The model under review builds one solid part; all positions refer to its coordinate system, in mm. A direction names the side the tool comes from. Coordinates: 2 decimals unless noted, no trailing zeros. Loops run counter-clockwise (first coordinate to the right, second up) from the corner with the lowest first, then second, coordinate; pieces in that order, holes last. Notation, with made-up numbers: M 35.5,20 L 93.5,20 A25 ccw 93.5,46 Z; hole C -17,24.5 d8. An arc over 180 degrees is marked long. Return JSON: item names as keys, results as strings.
```python
from build123d import *

# Parameters (mm, degrees)
F0_W     = 1000
F0_H     = 600
F1_DEPTH = 25
F2_W     = 960
F2_H     = 560
F3_DEPTH = 400
F4_W     = 940
F4_H     = 540
F5_DEPTH = 380
F6_W     = 25
F6_H     = 25
F7_DEPTH = 500
F8_R     = 25
F9_DEPTH = 100


with BuildPart() as f1:
    # F0 (on Top) → F1 (new body)
    with BuildSketch(Plane.XY):
        Rectangle(F0_W, F0_H)
    extrude(amount=F1_DEPTH)

    # F2 (on face) → F3 (join)
    with BuildSketch(Plane.XY.offset(25)):
        Rectangle(F2_W, F2_H)
    extrude(amount=F3_DEPTH)

    # F4 (on face) → F5 (cut)
    with BuildSketch(Plane(origin=(0, 0, 0), x_dir=(1, 0, 0), z_dir=(0, 0, -1))):
        Rectangle(F4_W, F4_H)
    extrude(amount=-F5_DEPTH, mode=Mode.SUBTRACT)

    # F6 (on face) → F7 (join)
    with BuildSketch(Plane.XY.offset(425)):
        with Locations((-467.5, 267.5)):
            Rectangle(F6_W, F6_H)
        with Locations((-467.5, -267.5)):
            Rectangle(F6_W, F6_H)
        with Locations((467.5, -267.5)):
            Rectangle(F6_W, F6_H)
        with Locations((467.5, 267.5)):
            Rectangle(F6_W, F6_H)
    extrude(amount=F7_DEPTH)

    # F8 (on face) → F9 (cut)
    with BuildSketch(Plane(origin=(0, 0, 380), x_dir=(1, 0, 0), z_dir=(0, 0, -1))):
        Circle(F8_R)
    extrude(amount=-F9_DEPTH, mode=Mode.SUBTRACT)


solid = f1.part
```
1. Add section B-B on z = 517. Give the boundary of the cut face in (x, y).
Check values:
{"outline": "M -480,-280 L -455,-280 L -455,-255 L -480,-255 Z; M -480,255 L -455,255 L -455,280 L -480,280 Z; M 455,-280 L 480,-280 L 480,-255 L 455,-255 Z; M 455,255 L 480,255 L 480,280 L 455,280 Z"}
2. Insertion check: pin 1 Ø7.5 at (x, z) = (-473, 627) entering from +Y; pin 2 Ø6 at (x, y) = (-204.5, 67) entering from -Z; pin 3 Ø12.5 at (x, z) = (472.5, 719.5) entering from -Y. Each pin has a flat end and moves straight along its axis. Give the tip position at first contact, or say it passes through.
Check values:
{"pin 1": "y = 280", "pin 2": "z = 380", "pin 3": "y = -280"}
3. To check wall thickness, follow line 1 (Y direction, x = 0, z = 390.5); line 2 (X direction, y = 47, z = 313); line 3 (Y direction, x = -145.5, z = 217.5). State the ranges of each line that lie inside material, in increasing order.
Check values:
{"line 1": "-280 to -25, 25 to 280", "line 2": "-480 to -470, 470 to 480", "line 3": "-280 to -270, 270 to 280"}
4. Add section A-A on y = 0. Give the boundary of the cut face in (x, z).
Check values:
{"outline": "M -500,0 L -470,0 L -470,380 L -25,380 L -25,425 L -480,425 L -480,25 L -500,25 Z; M 25,380 L 470,380 L 470,0 L 500,0 L 500,25 L 480,25 L 480,425 L 25,425 Z"}
5. The part is to be moulded in two halves that separate along Y. For faces 1 (the face through (467, 255, 672)), 2 (the face through (-7, 280, 169)), 3 (the face through (-39, -287, 0)), say which applies: released by +Y, released by -Y, zero draft, split by the parting line, or undercut.
Check values:
{"face 1": "undercut", "face 2": "released by +Y", "face 3": "zero draft"}
6. Add section D-D on z = 275. Give the boundary of the cut face in (x, y).
Check values:
{"outline": "M -480,-280 L 480,-280 L 480,280 L -480,280 Z; hole M -470,-270 L 470,-270 L 470,270 L -470,270 Z"}
7. Machinability: for faces 4 (the face through (-480, -4, 169)), 5 (the face through (-455, 267, 672)), 6 (the face through (-468, -267, 925)), 7 (the face through (-7, -64, 380)), 8 (the face through (-468, 255, 672)), which of the approach directions +Z, -Z, +X, -X, +Y, -Y give a long, thin tool a straight path to every point of the face, cutting with its end or side? Answer none if there is none.
Check values:
{"face 4": "+Z, -X, +Y, -Y", "face 5": "+Z, +Y, -Y", "face 6": "+Z, +X, -X, +Y, -Y", "face 7": "-Z", "face 8": "+Z, +X, -X"}
8. Add section C-C on x = 0. Give the boundary of the cut face in (y, z).
Check values:
{"outline": "M -300,0 L -270,0 L -270,380 L -25,380 L -25,425 L -280,425 L -280,25 L -300,25 Z; M 25,380 L 270,380 L 270,0 L 300,0 L 300,25 L 280,25 L 280,425 L 25,425 Z"}
